from build123d import *

# Parameters (mm, degrees)
SKETCH2_R           = 3.475
BOSS_EXTRUDE2_DEPTH = 30.6846
SKETCH3_R           = 1.475
CUT_EXTRUDE1_DEPTH  = 10
CUT_EXTRUDE2_START  = -10
SKETCH4_R           = 1.475
CUT_EXTRUDE2_DEPTH  = 10
BOSS_EXTRUDE3_DEPTH = 30.6846
SKETCH6_W           = 6.95
SKETCH6_H           = 30.6846
CUT_EXTRUDE3_DEPTH  = 0.3


with BuildPart() as part:
    # Sketch2 → Boss-Extrude2 (new body)
    with BuildSketch(Plane.XY):
        Circle(SKETCH2_R)
    extrude(amount=BOSS_EXTRUDE2_DEPTH)

    # Sketch3 → Cut-Extrude1 (cut)
    with BuildSketch(Plane.XY.offset(30.6846)):
        Circle(SKETCH3_R)
    extrude(amount=-CUT_EXTRUDE1_DEPTH, mode=Mode.SUBTRACT)

    # Sketch4 → Cut-Extrude2 (cut)
    with BuildSketch(Plane(origin=(0, 0, 0), x_dir=(-1, 0, 0), z_dir=(0, 0, -1)).offset(CUT_EXTRUDE2_START)):
        with Locations(Location((0, 0, 0), (0, 0, 180))):
            Circle(SKETCH4_R)
    extrude(amount=CUT_EXTRUDE2_DEPTH, mode=Mode.SUBTRACT)

    # Sketch5 → Boss-Extrude3 (add)
    with BuildSketch(Plane(origin=(0, 0, 0), x_dir=(-1, 0, 0), z_dir=(0, 0, -1))):
        with BuildLine():
            ThreePointArc((0, -3.475), (-2.457196065, -2.457196065), (-3.475, 0))
            Line((-3.475, 0), (-3.475, -3.475))
            Line((-3.475, -3.475), (0, -3.475))
        make_face()
        with BuildLine():
            Line((3.475, -3.475), (3.475, 0))
            ThreePointArc((3.475, 0), (2.457196065, -2.457196065), (0, -3.475))
            Line((0, -3.475), (3.475, -3.475))
        make_face()
    extrude(amount=-BOSS_EXTRUDE3_DEPTH)

    # Sketch6 → Cut-Extrude3 (cut)
    with BuildSketch(Plane(origin=(0, -3.475, 0), x_dir=(-1, 0, 0), z_dir=(0, -1, 0))):
        with Locations((0, -15.3423)):
            Rectangle(SKETCH6_W, SKETCH6_H)
    extrude(amount=-CUT_EXTRUDE3_DEPTH, mode=Mode.SUBTRACT)


solid = part.part
Can you work these out from the model? Positions are in its coordinate system, mm. A direction names the side the tool comes from. Give positions to 0.01 mm unless a question says otherwise; leave off trailing zeros. Order: outer loops, then holes, each group sorted by start corner. A loop starts at its lowest first (then second) coordinate and runs counter-clockwise, first axis right, second up. Notation, with made-up numbers: M 36,74 L 71,74 A17 ccw 71,105 Z; hole C 78,36.25 d10. An arc over 180 degrees is marked long. Use a Markdown table: item, result. Add a question column.
Item 1: We'd pull the mould along X, two halves only. Please class faces 4 (the flat face through (2, 0, 0)), 5 (the flat face through (0, 0, 10)), 6 (the flat face through (3.475, -2, 15)): +X half, -X half, draft (parallel to the pull), parting line (faces both ways), or undercut.
Item 2: Suppose I cut it at B-B (x = 0). List the corners of the cut face in (y, z) for me (3 decimals), then the cut area to 3 significant figures.
Item 3: Suppose I cut it at C-C (y = -0.75). List the corners of the cut face in (x, z) for me (3 decimals).
Item 4: If I drill on L1, parallel to Y at x = 0, z = 27 (3 decimals); L2, parallel to Z at x = 0, y = 1; L3, parallel to X at y = 1.25, z = 29, over which ranges is the centre line in solid material (lowest first)? Write a range as [from, to].
Item 5: Will these pins go through, and if not, where does the flat tip stop? pin 1 (1.5 mm diameter, centred on x = -2.5, z = 12.5, fed in from +Y); pin 2 (2.5 mm diameter, centred on x = 0, y = 0, fed in from -Z).
Item 6: For faces 1 (the flat face through (0, -3.175, 15)), 2 (the cylindrical face through (-1.474, 0.065, 25.755)), 3 (the cylindrical face through (-1.474, -0.065, 5.07)), which set-ups out of +Z, -Z, +X, -X, +Y, -Y let a thin tool reach every point of the face, with its end or its side?
Item 7: Suppose I cut it at D-D (z = 12.5). List the corners of the cut face in (x, y) for me (3 decimals).
Item 8: Suppose I cut it at A-A (z = 27). List the corners of the cut face in (x, y) for me (3 decimals), then the cut area to 3 significant figures.
Answer sheet:
| question | item | result |
|---|---|---|
| 1 | face 4 | draft |
| 1 | face 5 | undercut |
| 1 | face 6 | +X half |
| 2 | outline | M -3.175,0 L -1.475,0 L -1.475,10 L 1.475,10 L 1.475,0 L 3.475,0 L 3.475,30.685 L 1.475,30.685 L 1.475,20.685 L -1.475,20.685 L -1.475,30.685 L -3.175,30.685 Z |
| 2 | area | 145 mm² |
| 3 | outline | M -3.475,0 L -1.27,0 L -1.27,10 L 1.27,10 L 1.27,0 L 3.475,0 L 3.475,30.685 L 1.27,30.685 L 1.27,20.685 L -1.27,20.685 L -1.27,30.685 L -3.475,30.685 Z |
| 4 | L1 | y = [-3.175, -1.475], [1.475, 3.475] |
| 4 | L2 | z = [10, 20.68] |
| 4 | L3 | x = [-3.24, -0.78], [0.78, 3.24] |
| 5 | pin 1 | stops at y = 3 |
| 5 | pin 2 | stops at z = 10 |
| 6 | face 1 | +Z, -Z, +X, -X, -Y |
| 6 | face 2 | +Z |
| 6 | face 3 | -Z |
| 7 | outline | M -3.475,-3.175 L 3.475,-3.175 L 3.475,0 A3.475 ccw -3.475,0 Z |
| 8 | outline | M -3.475,-3.175 L 3.475,-3.175 L 3.475,0 A3.475 ccw -3.475,0 Z; hole C 0,0 d2.95 |
| 8 | area | 34.2 mm² |
